from build123d import *

# Parameters (mm, degrees)
ESQUISSE1_W              = 26
ESQUISSE1_H              = 50
BOSS_EXTRU_1_DEPTH       = 40
ESQUISSE2_W              = 20
ESQUISSE2_H              = 20
ENL_V_MAT_EXTRU_1_DEPTH  = 41
ESQUISSE3_W              = 6
ESQUISSE3_H              = 4
ESQUISSE3_W_2            = 4
ESQUISSE3_H_2            = 6
BOSS_EXTRU_2_DEPTH       = 40
ESQUISSE7_W              = 21
ESQUISSE7_H              = 20
ENL_V_MAT_EXTRU_4_DEPTH  = 41
ESQUISSE8_W              = 6
ESQUISSE8_H              = 2
ENL_V_MAT_EXTRU_5_DEPTH  = 41
ESQUISSE9_W              = 6
ESQUISSE9_H              = 4
ENL_V_MAT_EXTRU_6_DEPTH  = 3.5
ESQUISSE10_R             = 2.1
ENL_V_MAT_EXTRU_7_DEPTH  = 27
ENL_V_MAT_EXTRU_9_DEPTH  = 6
ESQUISSE13_W             = 26
ESQUISSE13_H             = 5
ENL_V_MAT_EXTRU_10_DEPTH = 41
CONG_1_R                 = 1
CONG_2_R                 = 1
ESQUISSE14_W             = 6
ESQUISSE14_H             = 40
BOSS_EXTRU_3_DEPTH       = 12
CHANFREIN1_SIZE          = 7
CHANFREIN1_SIZE2         = 4.041451884
CHANFREIN1_PART_2_SIZE   = 7
CHANFREIN1_PART_2_SIZE2  = 4.041451884
CONG_3_R                 = 2
ESQUISSE16_R             = 2.1
ENL_V_MAT_EXTRU_11_DEPTH = 27


with BuildPart() as part:
    # Esquisse1 → Boss.-Extru.1 (new body)
    with BuildSketch(Plane.XY):
        Rectangle(ESQUISSE1_W, ESQUISSE1_H)
    extrude(amount=BOSS_EXTRU_1_DEPTH)

    # Esquisse2 → Enlèv. mat.-Extru.1 (cut, through all)
    with BuildSketch(Plane.XY.offset(40)):
        with Locations((-3, -10)):
            Rectangle(ESQUISSE2_W, ESQUISSE2_H)
    extrude(amount=-ENL_V_MAT_EXTRU_1_DEPTH, mode=Mode.SUBTRACT)

    # Esquisse3 → Boss.-Extru.2 (add)
    with BuildSketch(Plane.XY.offset(40)):
        with Locations((-3, -2)):
            Rectangle(ESQUISSE3_W, ESQUISSE3_H)
        with Locations((5, -10)):
            Rectangle(ESQUISSE3_W_2, ESQUISSE3_H_2)
    extrude(amount=-BOSS_EXTRU_2_DEPTH)

    # Esquisse7 → Enlèv. mat.-Extru.4 (cut, through all)
    with BuildSketch(Plane.XY.offset(40)):
        with Locations((-2.5, 15)):
            Rectangle(ESQUISSE7_W, ESQUISSE7_H)
    extrude(amount=-ENL_V_MAT_EXTRU_4_DEPTH, mode=Mode.SUBTRACT)

    # Esquisse8 → Enlèv. mat.-Extru.5 (cut, through all)
    with BuildSketch(Plane.XY.offset(40)):
        with Locations((-3, 2.5)):
            Rectangle(ESQUISSE8_W, ESQUISSE8_H)
    extrude(amount=-ENL_V_MAT_EXTRU_5_DEPTH, mode=Mode.SUBTRACT)

    # Esquisse9 → Enlèv. mat.-Extru.6 (cut)
    with BuildSketch(Plane(origin=(0, 5, 0), x_dir=(1, 0, 0), z_dir=(0, 1, 0))):
        with Locations((-3, -33)):
            Rectangle(ESQUISSE9_W, ESQUISSE9_H)
        with Locations((-3, -7)):
            Rectangle(ESQUISSE9_W, ESQUISSE9_H)
    extrude(amount=-ENL_V_MAT_EXTRU_6_DEPTH, mode=Mode.SUBTRACT)

    # Esquisse10 → Enlèv. mat.-Extru.7 (cut, through all)
    with BuildSketch(Plane(origin=(13, 0, 0), x_dir=(0, 0, -1), z_dir=(1, 0, 0))):
        with Locations((-35, 18)):
            Circle(ESQUISSE10_R)
        with Locations((-5, 18)):
            Circle(ESQUISSE10_R)
    extrude(amount=-ENL_V_MAT_EXTRU_7_DEPTH, mode=Mode.SUBTRACT)

    # Esquisse12 → Enlèv. mat.-Extru.9 (cut, through all)
    with BuildSketch(Plane.ZY.offset(-8)):
        with BuildLine():
            Line((9, 13), (13, 13))
            ThreePointArc((13, 13), (20, 9.097518313), (27, 13))
            Line((27, 13), (31, 13))
            ThreePointArc((31, 13), (20, 7.247854519), (9, 13))
        make_face()
    extrude(amount=-ENL_V_MAT_EXTRU_9_DEPTH, mode=Mode.SUBTRACT)

    # Esquisse13 → Enlèv. mat.-Extru.10 (cut, through all)
    with BuildSketch(Plane(origin=(0, 0, 0), x_dir=(-1, 0, 0), z_dir=(0, 0, -1))):
        with Locations((0, -22.5)):
            Rectangle(ESQUISSE13_W, ESQUISSE13_H)
    extrude(amount=-ENL_V_MAT_EXTRU_10_DEPTH, mode=Mode.SUBTRACT)

    # Congé1
    cong_1_edges = [part.edges().sort_by_distance(p)[0] for p in [
        (-13, 0, 20),
        (-13, 5, 20),
    ]]
    fillet(cong_1_edges, radius=CONG_1_R)

    # Congé2
    cong_2_edges = [part.edges().sort_by_distance(p)[0] for p in [
        (10.5, 13, 31),
        (10.5, 13, 9),
        (10.5, 13, 13),
        (10.5, 13, 27),
    ]]
    fillet(cong_2_edges, radius=CONG_2_R)

    # Esquisse14 → Boss.-Extru.3 (add)
    with BuildSketch(Plane.XZ.offset(20)):
        with Locations((10, 20)):
            Rectangle(ESQUISSE14_W, ESQUISSE14_H)
    extrude(amount=BOSS_EXTRU_3_DEPTH)

    # Chanfrein1
    chanfrein1_edges = [part.edges().sort_by_distance(p)[0] for p in [
        (10.5, 25, 40),
        (10.5, 25, 0),
    ]]
    chanfrein1_side = [part.faces().sort_by_distance(p)[0] for p in [
        (10.5, 25, 20),
    ]]
    chamfer(chanfrein1_edges, length=CHANFREIN1_SIZE, length2=CHANFREIN1_SIZE2, reference=chanfrein1_side[0])

    # Chanfrein1 part 2
    chanfrein1_part_2_edges = [part.edges().sort_by_distance(p)[0] for p in [
        (10, -32, 40),
        (10, -32, 0),
    ]]
    chanfrein1_part_2_side = [part.faces().sort_by_distance(p)[0] for p in [
        (10, -32, 20),
    ]]
    chamfer(chanfrein1_part_2_edges, length=CHANFREIN1_PART_2_SIZE, length2=CHANFREIN1_PART_2_SIZE2, reference=chanfrein1_part_2_side[0])

    # Congé3
    cong_3_edges = [part.edges().sort_by_distance(p)[0] for p in [
        (10, -32, 7),
        (10, -32, 33),
        (10.5, 20.958548116, 40),
        (10, -27.958548116, 40),
        (10.5, 20.958548116, 0),
        (10, -27.958548116, 0),
        (10.5, 25, 7),
        (10.5, 25, 33),
    ]]
    fillet(cong_3_edges, radius=CONG_3_R)

    # Esquisse16 → Enlèv. mat.-Extru.11 (cut, through all)
    with BuildSketch(Plane(origin=(13, 0, 0), x_dir=(0, 0, -1), z_dir=(1, 0, 0))):
        with Locations((-20, -27)):
            Circle(ESQUISSE16_R)
    extrude(amount=-ENL_V_MAT_EXTRU_11_DEPTH, mode=Mode.SUBTRACT)


solid = part.part
The model under review builds one solid part; all positions refer to its coordinate system, in mm. A direction names the side the tool comes from. Coordinates: 2 decimals unless noted, no trailing zeros. Loops run counter-clockwise (first coordinate to the right, second up) from the corner with the lowest first, then second, coordinate; pieces in that order, holes last. Notation, with made-up numbers: M 78,62 L 128,62 A27 ccw 128,83 Z; hole C 65.5,32 d10. An arc over 180 degrees is marked long. Put each result on its own line as item: value. Start each with the question number.
Q1. Add section B-B (y = 2.5). Write out the cut boundary in (x, z).
Q2. Wall thickness on line 1 (Y direction, x = -4.75, z = 24); line 2 (X direction, y = 2, z = 35); line 3 (X direction, y = -2, z = 6.5): over which ranges is each line inside the solid? List them lowest first.
Q3. Add section A-A (z = 20). Count the separate pieces of the cut face and the enclosed holes in it, and give its area (3 significant figures).
Q4. The part is to be moulded in two halves that separate along X. For faces 6 (the flat face through (-6, 3, 20)), 7 (the flat face through (7, -22, 20)), 8 (the flat face through (13, -3, 20)), 9 (the cylindrical face through (10.5, 9.1, 19.9)), say which applies: +X half, -X half, draft (parallel to the pull), parting line (faces both ways), or undercut.
Q5. For faces 1 (the flat face through (3, -10, 20)), 2 (the flat face through (-3, 4, 31)), 3 (the flat face through (5, -7, 20)), 4 (the cylindrical face through (10.5, 12.4, 10.2)), 5 (the flat face through (-3, 3.5, 20)), list the 3-axis set-ups (+Z, -Z, +X, -X, +Y, -Y) from which the entire face can be reached by the end or side of a thin tool; tool diameter is ignored.
Q6. Add section C-C (x = -1.5). Write out the cut boundary in (y, z), and give its area (3 significant figures).
Q7. Add section D-D (z = 24). Write out the cut boundary in (x, y), and give its area (3 significant figures).
Q8. Clearance check with flat-ended pins moving along their axes: pin 1 (5.5 mm diameter, centred on y = -3.5, z = 24.5, fed in from -X); pin 2 (5.5 mm diameter, centred on x = -3.5, z = 3, fed in from -Y); pin 3 (5 mm diameter, centred on x = -9, z = 10.5, fed in from -Y); pin 4 (1.5 mm diameter, centred on x = 1, y = -12, fed in from -Z). State where each tip first meets the part, or that it passes through.
Answers:
1. outline: M -13,0 L -6,0 L -6,40 L -13,40 Z; M 0,0 L 13,0 L 13,40 L 0,40 Z
2. line 1: y = -4 to 1.5, 3.5 to 5
2. line 2: x = -13 to -6, 0 to 13
2. line 3: x = -6 to 0, 7 to 13
3. separate pieces: 3
3. enclosed holes: 1
3. area: 423 mm^2
4. face 6: undercut
4. face 7: -X half
4. face 8: +X half
4. face 9: draft
5. face 1: +Z, -Z, -X, -Y
5. face 2: +Y
5. face 3: +Z, -Z, -X
5. face 4: +X, -X
5. face 5: +Z, -Z
6. outline: M -4,0 L 1.5,0 L 1.5,40 L -4,40 Z; M 3.5,0 L 5,0 L 5,5 L 3.5,5 Z; M 3.5,9 L 5,9 L 5,31 L 3.5,31 Z; M 3.5,35 L 5,35 L 5,40 L 3.5,40 Z
6. area: 268 mm^2
7. outline: M -13,1 A1 ccw -12,0 L -6,0 L -6,-4 L 0,-4 L 0,0 L 7,0 L 7,-7 L 3,-7 L 3,-13 L 7,-13 L 7,-32 L 13,-32 L 13,7.86 L 8,7.86 L 8,5 L -12,5 A1 ccw -13,4 Z; M 8,10.14 L 13,10.14 L 13,25 L 8,25 Z; hole M -6,1.5 L 0,1.5 L 0,3.5 L -6,3.5 Z
7. area: 446 mm^2
8. pin 1: stops at x = -6
8. pin 2: stops at y = -4
8. pin 3: stops at y = 0
8. pin 4: passes through
